from build123d import *

# Parameters (mm, degrees)
FRAME_EXTERIOR_MASTER_OUTLINE_R = 19.685
FRAME_EXTERIOR_MASTER_DEPTH     = 6.35
SKETCH1_R                       = 1.75
CUT_EXTRUDE1_DEPTH              = 611.690430988


# Read off the part's stored shape, not the designer's step: Frame Exterior Master
with BuildPart() as part:
    # Frame Exterior Master outline → Frame Exterior Master (new body)
    with BuildSketch(Plane.XY):
        Polygon((431.8, 12.7), (431.8, 431.8), (215.9, 431.8), (0, 304.8), (0, 12.7), (127, 12.7), (127, 50.8), (254, 50.8), (254, 12.7), align=None)
        with Locations((98.15, 150.3)):
            Circle(FRAME_EXTERIOR_MASTER_OUTLINE_R, mode=Mode.SUBTRACT)
        with Locations((333.65, 150.3)):
            Circle(FRAME_EXTERIOR_MASTER_OUTLINE_R, mode=Mode.SUBTRACT)
    extrude(amount=FRAME_EXTERIOR_MASTER_DEPTH)

    # Sketch1 → Cut-Extrude1 (cut, through all)
    with BuildSketch(Plane.XY.offset(6.35)):
        with Locations((316.667678943, 38.1)):
            Circle(SKETCH1_R)
    extrude(amount=-CUT_EXTRUDE1_DEPTH, mode=Mode.SUBTRACT)


solid = part.part
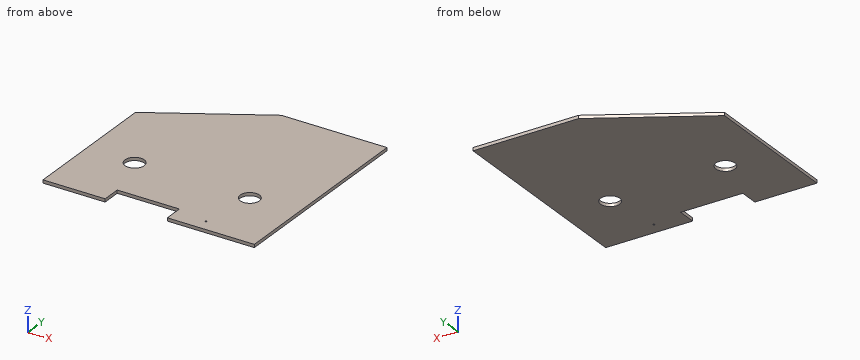
Could you check a few things on this model? Use its own coordinates, in mm. Give positions to 0.01 mm unless a question says otherwise; leave off trailing zeros. Write each loop counter-clockwise with the first axis right and the second up, starting at its lowest first coordinate (ties: lowest second). Pieces come first, ordered by that corner, then holes. Notation, with made-up numbers: (20.25, 79) -> (25.25, 79) arc R19 ccw to (25.25, 88) -> close; hole circle Ø4 at (-17.5, 19). An arc over 180 degrees is marked (long way). Answer as CSV lines item,"result". Start each with the question number.
(1) If we section it at B-B, the plane z = 5: Write out the boundary of the cut face in (x, y) (3 decimals).
(2) If we section it at A-A, the plane y = 150.3: Write out the boundary of the cut face in (x, z) (3 decimals).
(3) If we section it at C-C, the plane x = 333.65: Write out the boundary of the cut face in (y, z) (3 decimals), and give its area (3 significant figures).
(4) Please list where these lines run through material, in increasing order: line 1 (Y direction, x = 333.65, z = 3.25) (3 decimals); line 2 (Y direction, x = 98.15, z = 2.5) (3 decimals); line 3 (Y direction, x = 225.5, z = 1.5).
(5) If we section it at D-D, the plane x = 143: Write out the boundary of the cut face in (y, z).
(6) I'm going to push flat-ended pins straight in: pin 1 Ø3 at (x, z) = (208, 4.5) entering from -Y; pin 2 Ø3 at (x, y) = (316.67, 38.1) entering from +Z. Where does each tip first touch, or does it pass through?
Answer list:
1,outline,"(0, 12.7) -> (127, 12.7) -> (127, 50.8) -> (254, 50.8) -> (254, 12.7) -> (431.8, 12.7) -> (431.8, 431.8) -> (215.9, 431.8) -> (0, 304.8) -> close; hole circle Ø39.37 at (98.15, 150.3); hole circle Ø39.37 at (333.65, 150.3); hole circle Ø3.5 at (316.668, 38.1)"
2,outline,"(0, 0) -> (78.465, 0) -> (78.465, 6.35) -> (0, 6.35) -> close; (117.835, 0) -> (313.965, 0) -> (313.965, 6.35) -> (117.835, 6.35) -> close; (353.335, 0) -> (431.8, 0) -> (431.8, 6.35) -> (353.335, 6.35) -> close"
3,outline,"(12.7, 0) -> (130.615, 0) -> (130.615, 6.35) -> (12.7, 6.35) -> close; (169.985, 0) -> (431.8, 0) -> (431.8, 6.35) -> (169.985, 6.35) -> close"
3,area,"2,410 mm^2"
4,line 1,"12.7 to 130.615, 169.985 to 431.8"
4,line 2,"12.7 to 130.615, 169.985 to 362.535"
4,line 3,"50.8 to 431.8"
5,outline,"(50.8, 0) -> (388.92, 0) -> (388.92, 6.35) -> (50.8, 6.35) -> close"
6,pin 1,"y = 50.8"
6,pin 2,"through"
